Part print with two shaded views. Sizes in mm from the minimum x, y, z corner. A direction names the side the tool comes from. Give positions to 0.01 mm unless a question says otherwise; leave off trailing zeros. Loops run counter-clockwise (first coordinate to the right, second up) from the corner with the lowest first, then second, coordinate; pieces in that order, holes last. Notation, with made-up numbers: M 81.5,86.25 L 113.5,86.25 A27 cw 113.5,118.25 Z; hole C -0.75,0 d4. An arc over 180 degrees is marked long. Answer as a JSON object with one key per item and string values. Group by question number.
1. Mould opens along X. For the marked faces 1, 2 and 3 say: released by +X, released by -X, zero draft, split by the parting line, or undercut.
2. Slice it at B-B (z = 1). List the corners of the cut face in (x, y) (3 decimals).
3. Drill centre lines: line 1 along Y through (x, z) = (19.5, 2); line 2 along Y through (x, z) = (14.5, 5.75); line 3 along X through (y, z) = (6, 2.5). Where is each one in solid material? Low to high. Write a range as [from, to].
4. Slice it at C-C (y = 16). List the corners of the cut face in (x, z) (3 decimals), then the cut area to 3 significant figures.
5. Slice it at D-D (x = 3). List the corners of the cut face in (y, z), then the cut area to 3 significant figures.
6. 3-axis set-ups, long thin cutter, end or side, ignore diameter. For the marked faces 4, 5, 6 and 7: which of +Z, -Z, +X, -X, +Y, -Y reach the whole face in a straight line?
7. Slice it at A-A (y = 35.5). List the corners of the cut face in (x, z) (3 decimals).
8. Drop flat-ended pins along their axis: pin 1 Ø3 at (y, z) = (35, 3.5) entering from -X; pin 2 Ø3 at (y, z) = (8, 4) entering from +X; pin 3 Ø6 at (x, y) = (16.5, 16.5) entering from -Z; pin 4 Ø1.9 at (x, z) = (9.5, 2) entering from -Y. Give the stop position or say it passes through.
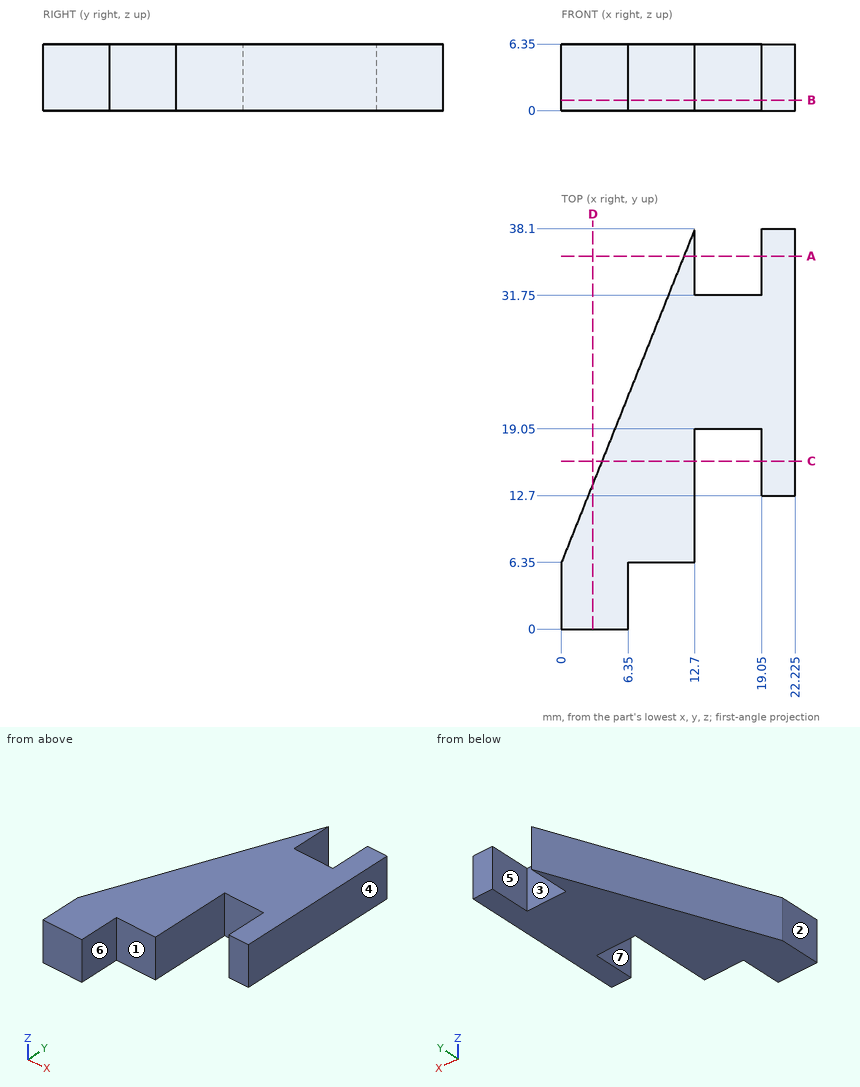
Established:
{
 "1": {"face 1": "zero draft", "face 2": "released by -X", "face 3": "undercut"},
 "2": {"outline": "M 0,0 L 6.35,0 L 6.35,6.35 L 12.7,6.35 L 12.7,19.05 L 19.05,19.05 L 19.05,12.7 L 22.225,12.7 L 22.225,38.1 L 19.05,38.1 L 19.05,31.75 L 12.7,31.75 L 12.7,38.1 L 0,6.35 Z"},
 "3": {"line 1": "y = [12.7, 38.1]", "line 2": "y = [19.05, 31.75]", "line 3": "x = [0, 6.35]"},
 "4": {"outline": "M 3.86,0 L 12.7,0 L 12.7,6.35 L 3.86,6.35 Z; M 19.05,0 L 22.225,0 L 22.225,6.35 L 19.05,6.35 Z", "area": "76.3 mm^2"},
 "5": {"outline": "M 0,0 L 13.85,0 L 13.85,6.35 L 0,6.35 Z", "area": "87.9 mm^2"},
 "6": {"face 4": "+Z, -Z, +X, +Y, -Y", "face 5": "+Z, -Z, +Y", "face 6": "+Z, -Z, +X, -Y", "face 7": "+Z, -Z, -Y"},
 "7": {"outline": "M 11.66,0 L 12.7,0 L 12.7,6.35 L 11.66,6.35 Z; M 19.05,0 L 22.225,0 L 22.225,6.35 L 19.05,6.35 Z"},
 "8": {"pin 1": "stops at x = 10.86", "pin 2": "stops at x = 12.7", "pin 3": "stops at z = 0", "pin 4": "stops at y = 6.35"}
}
